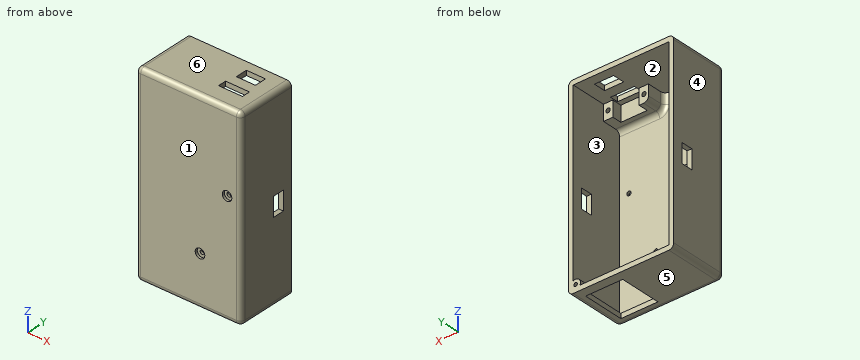
from build123d import *
from build123d.topology import SkipClean

# Parameters (mm, degrees)
SKETCH_1_W           = 44
SKETCH_1_H           = 81
EXTRUDE_1_DEPTH      = 25
SHELL_1_T            = -2
FILLET_1_R           = 2
SKETCH_2_R           = 0.8
SKETCH_2_R_2         = 0.9
CUT_EXTRUDE_1_DEPTH  = 24
SKETCH_3_R           = 1.25
CUT_EXTRUDE_2_DEPTH  = 24
SKETCH_4_R           = 6
EXTRUDE_2_DEPTH      = 2
CUT_EXTRUDE_START    = -13.2
SKETCH_6_R           = 1.25
CUT_EXTRUDE_4_DEPTH  = 13.2
SKETCH_7_W           = 15.5
SKETCH_7_H           = 17.5
CUT_EXTRUDE_5_DEPTH  = 13.2
SKETCH_9_W           = 18.8
SKETCH_9_H           = 6.5
SKETCH_9_R           = 0.9
EXTRUDE_3_DEPTH      = 8
SKETCH_11_W          = 11
SKETCH_11_H          = 6.5
CUT_EXTRUDE_6_DEPTH  = 4
SKETCH_12_W          = 10
SKETCH_12_H          = 3.5
CUT_EXTRUDE_7_DEPTH  = 4
FILLET_2_R           = 2
EXTRUDE_START        = -1
SKETCH_14_R          = 1.25
EXTRUDE_4_DEPTH      = 1
SKETCH_15_R          = 2
CUT_EXTRUDE_8_DEPTH  = 1
SKETCH_16_W          = 8
SKETCH_16_H          = 5
CUT_EXTRUDE_9_DEPTH  = 59
SKETCH_17_R          = 2
EXTRUDE_5_DEPTH      = 3
SKETCH_18_R          = 0.75
CUT_EXTRUDE_10_DEPTH = 3
FILLET_3_R           = 2
SKETCH_19_W          = 8
SKETCH_19_H          = 5
CUT_EXTRUDE_11_DEPTH = 3


with BuildPart() as part:
    # 草图1 → 凸台-拉伸1 (new body)
    with BuildSketch(Plane(origin=(0, 0, 0), x_dir=(1, 0, 0), z_dir=(0, 1, 0))):
        with Locations((0, -2.5)):
            Rectangle(SKETCH_1_W, SKETCH_1_H)
    extrude(amount=EXTRUDE_1_DEPTH)

    # 抽壳1
    shell_1_openings = [part.faces().sort_by_distance(p)[0] for p in [
        (0, 25, 2.5),
    ]]
    offset(amount=SHELL_1_T, openings=shell_1_openings, kind=Kind.INTERSECTION)

    # 圆角1
    fillet_1_edges = [part.edges().sort_by_distance(p)[0] for p in [
        (0, 0, -38),
        (22, 0, 2.5),
        (0, 0, 43),
        (-22, 0, 2.5),
        (-22, 12.5, -38),
        (22, 12.5, -38),
        (22, 12.5, 43),
        (-22, 12.5, 43),
    ]]
    fillet(fillet_1_edges, radius=FILLET_1_R)

    # 草图2 → 切除-拉伸1 (cut)
    with BuildSketch(Plane(origin=(0, 2, 0), x_dir=(1, 0, 0), z_dir=(0, 1, 0))):
        with Locations(Location((4.8, 16.9, 0), (0, 0, 270))):
            Circle(SKETCH_2_R)
        with Locations(Location((16.1, -9.5, 0), (0, 0, 270))):
            Circle(SKETCH_2_R_2)
    extrude(amount=-CUT_EXTRUDE_1_DEPTH, mode=Mode.SUBTRACT)

    # 草图3 → 切除-拉伸2 (cut)
    with BuildSketch(Plane(origin=(0, 2, 0), x_dir=(1, 0, 0), z_dir=(0, 1, 0))):
        with Locations(Location((-9.5, -3, 0), (0, 0, 270))):
            Circle(SKETCH_3_R)
    extrude(amount=-CUT_EXTRUDE_2_DEPTH, mode=Mode.SUBTRACT)

    # 草图4 → 凸台-拉伸2 (add)
    with BuildSketch(Plane(origin=(0, 2, 0), x_dir=(1, 0, 0), z_dir=(0, 1, 0))):
        with Locations(Location((-9.5, -3, 0), (0, 0, 270))):
            Circle(SKETCH_4_R)
    extrude(amount=EXTRUDE_2_DEPTH)

    # 草图6 → 切除-拉伸4 (cut)
    with BuildSketch(Plane.XZ.offset(CUT_EXTRUDE_START)):
        with Locations(Location((-9.5, 3, 0), (0, 0, 90))):
            Circle(SKETCH_6_R)
    extrude(amount=CUT_EXTRUDE_4_DEPTH, mode=Mode.SUBTRACT)

    # 草图7 → 切除-拉伸5 (cut)
    with BuildSketch(Plane(origin=(0, 0, -38), x_dir=(-1, 0, 0), z_dir=(0, 0, -1))):
        with Locations((-10.25, 12.5)):
            Rectangle(SKETCH_7_W, SKETCH_7_H)
    extrude(amount=-CUT_EXTRUDE_5_DEPTH, mode=Mode.SUBTRACT)

    # 草图9 → 凸台-拉伸3 (add)
    with BuildSketch(Plane(origin=(0, 2, 0), x_dir=(1, 0, 0), z_dir=(0, 1, 0))):
        with Locations((10.6, -37.75)):
            Rectangle(SKETCH_9_W, SKETCH_9_H)
        with Locations(Location((18.1, -37.9, 0), (0, 0, 270))):
            Circle(SKETCH_9_R, mode=Mode.SUBTRACT)
        with Locations(Location((3.1, -37.9, 0), (0, 0, 270))):
            Circle(SKETCH_9_R, mode=Mode.SUBTRACT)
    extrude(amount=EXTRUDE_3_DEPTH)

    # 草图11 → 切除-拉伸6 (cut)
    with BuildSketch(Plane(origin=(0, 10, 0), x_dir=(1, 0, 0), z_dir=(0, 1, 0))):
        with Locations((10.6, -37.75)):
            Rectangle(SKETCH_11_W, SKETCH_11_H)
    extrude(amount=-CUT_EXTRUDE_6_DEPTH, mode=Mode.SUBTRACT)

    # 草图12 → 切除-拉伸7 (cut)
    with BuildSketch(Plane.XY.offset(43)):
        with Locations((10.6, 10)):
            Rectangle(SKETCH_12_W, SKETCH_12_H)
    extrude(amount=-CUT_EXTRUDE_7_DEPTH, mode=Mode.SUBTRACT)

    # 圆角2
    fillet_2_edges = [part.edges().sort_by_distance(p)[0] for p in [
        (10.6, 2, 34.5),
        (1.2, 2, 37.75),
        (1.2, 6, 34.5),
    ]]
    fillet(fillet_2_edges, radius=FILLET_2_R)

    # 草图14 → 凸台-拉伸4 (add)
    with BuildSketch(Plane.XZ.offset(EXTRUDE_START)):
        with Locations(Location((-9.5, 3, 0), (0, 0, 90))):
            Circle(SKETCH_14_R)
    extrude(amount=EXTRUDE_4_DEPTH)

    # 草图15 → 切除-拉伸8 (cut)
    with BuildSketch(Plane.XZ):
        with Locations(Location((16.1, 9.5, 0), (0, 0, 270))):
            Circle(SKETCH_15_R)
        with Locations(Location((4.8, -16.9, 0), (0, 0, 270))):
            Circle(SKETCH_15_R)
    extrude(amount=-CUT_EXTRUDE_8_DEPTH, mode=Mode.SUBTRACT)

    # 草图16 → 切除-拉伸9 (cut)
    with BuildSketch(Plane.ZY.offset(22)):
        with Locations((0, 18.5)):
            Rectangle(SKETCH_16_W, SKETCH_16_H)
    extrude(amount=-CUT_EXTRUDE_9_DEPTH, mode=Mode.SUBTRACT)

    # 草图17 → 凸台-拉伸5 (add)
    with BuildSketch(Plane(origin=(0, 25, 0), x_dir=(1, 0, 0), z_dir=(0, 1, 0))):
        with Locations((19, 35)):
            Circle(SKETCH_17_R)
    extrude(amount=-EXTRUDE_5_DEPTH)

    # 草图18 → 切除-拉伸10 (cut)
    with BuildSketch(Plane(origin=(0, 25, 0), x_dir=(1, 0, 0), z_dir=(0, 1, 0))):
        with Locations(Location((19, 35, 0), (0, 0, 270))):
            Circle(SKETCH_18_R)
    extrude(amount=-CUT_EXTRUDE_10_DEPTH, mode=Mode.SUBTRACT)

    # 圆角3
    # the kernel refuses this fillet: 2 mm, written as the material it adds along each edge
    with BuildSketch(Plane(origin=(12.267949192, 22, -36), x_dir=(0, -1, 0), z_dir=(1, 0, 0))) as fillet_3_piece_1_section:
        with BuildLine():
            CenterArc((FILLET_3_R, -FILLET_3_R), FILLET_3_R, 90, 90)
            Line((0, -FILLET_3_R), (0, 0))
            Line((0, 0), (FILLET_3_R, 0))
        make_face()
    fillet_3_piece_1 = extrude(amount=7.732050808, mode=Mode.PRIVATE)
    fillet_3_piece_1 = fillet_3_piece_1 & Plane(origin=(19, 21.743486993, -35), x_dir=(1, 0, 0), z_dir=(0, 1, 0)) * Cylinder(2, 24, mode=Mode.PRIVATE)
    fillet_3_piece_1 = split(fillet_3_piece_1, bisect_by=Plane(origin=(18, 21.743486993, -35.418577815), z_dir=(-1, 0, 0)), keep=Keep.TOP, mode=Mode.PRIVATE)
    fillet_3_piece_1 = split(fillet_3_piece_1, bisect_by=Plane(origin=(17.546708028, 21.25, -35.418577815), z_dir=(0, 1, 0)), keep=Keep.TOP, mode=Mode.PRIVATE)
    add(fillet_3_piece_1)
    with BuildSketch(Plane(origin=(12.267949192, 22, -36), x_dir=(0, -1, 0), z_dir=(1, 0, 0))) as fillet_3_piece_2_section:
        with BuildLine():
            CenterArc((FILLET_3_R, -FILLET_3_R), FILLET_3_R, 90, 90)
            Line((0, -FILLET_3_R), (0, 0))
            Line((0, 0), (FILLET_3_R, 0))
        make_face()
    fillet_3_piece_2 = extrude(amount=7.732050808, mode=Mode.PRIVATE)
    fillet_3_piece_2 = split(fillet_3_piece_2, bisect_by=Plane(origin=(18, 20.864048259, -35.911747477), z_dir=(1, 0, 0)), keep=Keep.TOP, mode=Mode.PRIVATE)
    fillet_3_piece_2 = split(fillet_3_piece_2, bisect_by=Plane(origin=(18.99999999, 21.25, -35.911747477), z_dir=(0, -1, 0)), keep=Keep.TOP, mode=Mode.PRIVATE)
    fillet_3_piece_2 = fillet_3_piece_2 - Plane(origin=(19, 20.864048259, -35), x_dir=(0, 0, 1), z_dir=(0, 1, 0)) * Cylinder(0.75, 24, mode=Mode.PRIVATE)
    add(fillet_3_piece_2)
    with BuildSketch(Plane(origin=(12.267949192, 22, -36), x_dir=(0, -1, 0), z_dir=(1, 0, 0))) as fillet_3_piece_3_section:
        with BuildLine():
            CenterArc((FILLET_3_R, -FILLET_3_R), FILLET_3_R, 90, 90)
            Line((0, -FILLET_3_R), (0, 0))
            Line((0, 0), (FILLET_3_R, 0))
        make_face()
    fillet_3_piece_3 = extrude(amount=7.732050808, mode=Mode.PRIVATE)
    fillet_3_piece_3 = split(fillet_3_piece_3, bisect_by=Plane(origin=(18, 21.475531477, -35.364676357), z_dir=(1, 0, 0)), keep=Keep.TOP, mode=Mode.PRIVATE)
    fillet_3_piece_3 = split(fillet_3_piece_3, bisect_by=Plane(origin=(19.666666667, 21.25, -35.364676357), z_dir=(0, 1, 0)), keep=Keep.TOP, mode=Mode.PRIVATE)
    fillet_3_piece_3 = fillet_3_piece_3 - Plane(origin=(19, 21.475531477, -35), x_dir=(0, 0, 1), z_dir=(0, 1, 0)) * Cylinder(0.75, 24, mode=Mode.PRIVATE)
    add(fillet_3_piece_3)
    with BuildSketch(Plane(origin=(12.267949192, 22, -36), x_dir=(0, -1, 0), z_dir=(1, 0, 0))) as fillet_3_piece_4_section:
        with BuildLine():
            CenterArc((FILLET_3_R, -FILLET_3_R), FILLET_3_R, 90, 90)
            Line((0, -FILLET_3_R), (0, 0))
            Line((0, 0), (FILLET_3_R, 0))
        make_face()
    fillet_3_piece_4 = extrude(amount=12.732050808, mode=Mode.PRIVATE)
    fillet_3_piece_4 = split(fillet_3_piece_4, bisect_by=Plane(origin=(20, 20.885178509, -35.897350533), z_dir=(1, 0, 0)), keep=Keep.TOP, mode=Mode.PRIVATE)
    fillet_3_piece_4 = fillet_3_piece_4 & Plane(origin=(19, 20.885178509, -35), x_dir=(1, 0, 0), z_dir=(0, 1, 0)) * Cylinder(2, 34, mode=Mode.PRIVATE)
    fillet_3_piece_4 = split(fillet_3_piece_4, bisect_by=Plane(origin=(20.391607497, 21.25, -35.897350533), z_dir=(0, -1, 0)), keep=Keep.TOP, mode=Mode.PRIVATE)
    add(fillet_3_piece_4)
    with BuildSketch(Plane(origin=(12.267949192, 22, -36), x_dir=(0, -1, 0), z_dir=(1, 0, 0))) as fillet_3_piece_5_section:
        with BuildLine():
            CenterArc((FILLET_3_R, -FILLET_3_R), FILLET_3_R, 90, 90)
            Line((0, -FILLET_3_R), (0, 0))
            Line((0, 0), (FILLET_3_R, 0))
        make_face()
    fillet_3_piece_5 = extrude(amount=12.732050808, mode=Mode.PRIVATE)
    fillet_3_piece_5 = split(fillet_3_piece_5, bisect_by=Plane(origin=(20, 21.743487033, -35.418577693), z_dir=(1, 0, 0)), keep=Keep.TOP, mode=Mode.PRIVATE)
    fillet_3_piece_5 = fillet_3_piece_5 & Plane(origin=(19, 21.743487033, -35), x_dir=(1, 0, 0), z_dir=(0, 1, 0)) * Cylinder(2, 34, mode=Mode.PRIVATE)
    fillet_3_piece_5 = split(fillet_3_piece_5, bisect_by=Plane(origin=(20.45329205, 21.25, -35.418577693), z_dir=(0, 1, 0)), keep=Keep.TOP, mode=Mode.PRIVATE)
    add(fillet_3_piece_5)
    with BuildSketch(Plane(origin=(20, 22, -41), x_dir=(0, -1, 0), z_dir=(0, 0, 1))) as fillet_3_piece_6_section:
        with BuildLine():
            CenterArc((FILLET_3_R, -FILLET_3_R), FILLET_3_R, 90, 90)
            Line((0, -FILLET_3_R), (0, 0))
            Line((0, 0), (FILLET_3_R, 0))
        make_face()
    fillet_3_piece_6 = extrude(amount=12.732050808, mode=Mode.PRIVATE)
    fillet_3_piece_6 = fillet_3_piece_6 & Plane(origin=(19, 21.575046731, -35), x_dir=(1, 0, 0), z_dir=(0, 1, 0)) * Cylinder(2, 34, mode=Mode.PRIVATE)
    fillet_3_piece_6 = fillet_3_piece_6 - Plane(origin=(19, 21.575046731, -35), x_dir=(0, 0, 1), z_dir=(0, 1, 0)) * Cylinder(0.75, 34, mode=Mode.PRIVATE)
    add(fillet_3_piece_6)

    # 草图19 → 切除-拉伸11 (cut)
    with SkipClean():  # the faces are left unmerged after this step: merging them gives an invalid solid
        with BuildSketch(Plane.XY.offset(43)):
            with Locations((10.5, 18.5)):
                Rectangle(SKETCH_19_W, SKETCH_19_H)
        extrude(amount=-CUT_EXTRUDE_11_DEPTH, mode=Mode.SUBTRACT)


solid = part.part
Geometry check sheet. Reference: the model listing, model coordinates, mm. Face numbers are marked on the shaded views. A direction names the side the tool comes from. Round coordinates to 2 decimals unless told otherwise and drop trailing zeros. Write each loop counter-clockwise with the first axis right and the second up, starting at its lowest first coordinate (ties: lowest second). Pieces come first, ordered by that corner, then holes. Notation, with made-up numbers: (58.25, -34) - (94.25, -34) arc R25 cw to (94.25, -6) - close; hole circle Ø10 at (29.25, -7.5). An arc over 180 degrees is marked (long way). One line per item, written item: value.
1. Mould release check, pull along Z, two halves, no side actions. Record for the marked faces 3, 4, 5 and 6: released by +Z, released by -Z, zero draft, split by the parting line, or undercut.
The answers:
face 3: undercut
face 4: zero draft
face 5: released by -Z
face 6: released by +Z
2. Scan lines: L1, parallel to X at y = 22.9, z = -35; L2, parallel to Z at x = 19, y = 23.4; L3, parallel to X at y = 8.25, z = 37.9. Record each from-to range of solid material in increasing order.
The answers:
L1: x = -22 to -20, 17 to 18.25, 19.75 to 22
L2: z = -38 to -35.75, -34.25 to -33, 41 to 43
L3: x = -22 to -20, 1.2 to 2.2, 4 to 5.1, 16.1 to 17.2, 19 to 22
3. Cross-section at C-C on z = -16.9. Record the boundary of the cut face in (x, y).
The answers:
outline: (-22, 2) arc R2 ccw to (-20, 0) - (2.8, 0) - (2.8, 1) - (4, 1) - (4, 2) - (-20, 2) - (-20, 25) - (-22, 25) - close; (5.6, 1) - (6.8, 1) - (6.8, 0) - (20, 0) arc R2 ccw to (22, 2) - (22, 25) - (20, 25) - (20, 2) - (5.6, 2) - close
4. Set-up check for the marked faces 1 and 2: record each of +Z, -Z, +X, -X, +Y, -Y from which the full face is reachable in a straight line by a thin tool's end or side.
The answers:
face 1: +Z, -Z, +X, -X, -Y
face 2: +Y
5. Cross-section at B-B on x = 12. Record the boundary of the cut face in (y, z), and give its area (3 significant figures).
The answers:
outline: (0, -36) arc R2 ccw to (2, -38) - (3.75, -38) - (3.75, -36) - (2, -36) - (2, 32.5) arc R2 cw to (4, 34.5) - (6, 34.5) - (6, 41) - (8.25, 41) - (8.25, 43) - (2, 43) arc R2 ccw to (0, 41) - close; (11.75, 41) - (16, 41) - (16, 43) - (11.75, 43) - close; (21, 41) - (25, 41) - (25, 43) - (21, 43) - close; (21.25, -38) - (25, -38) - (25, -36) - (21.25, -36) - close
area: 227 mm^2
6. Cross-section at D-D on z = 37.9. Record the boundary of the cut face in (x, y), and give its area (3 significant figures).
The answers:
outline: (-22, 2) arc R2 ccw to (-20, 0) - (20, 0) arc R2 ccw to (22, 2) - (22, 25) - (20, 25) - (20, 10) - (19, 10) - (19, 2) - (17.2, 2) - (17.2, 10) - (16.1, 10) - (16.1, 6) - (5.1, 6) - (5.1, 10) - (4, 10) - (4, 2) - (2.2, 2) - (2.2, 10) - (1.2, 10) - (1.2, 4) arc R2 cw to (-0.8, 2) - (-20, 2) - (-20, 25) - (-22, 25) - close
area: 257 mm^2
7. Depth check by flat-ended pin: pin 1 Ø0.6 at (x, z) = (-21, 0) entering from -Y; pin 2 Ø1.6 at (y, z) = (12.5, -37) entering from +X; pin 3 Ø6 at (x, z) = (0, 25) entering from +Y; pin 4 Ø1 at (x, z) = (4.8, -16.9) entering from +Y. Enter the tip coordinate at first touch or a pass-through.
The answers:
pin 1: stops at y = 0.13
pin 2: stops at x = 21.99
pin 3: stops at y = 2
pin 4: passes through
8. Cross-section at A-A on y = 18.5. Record the boundary of the cut face in (x, z).
The answers:
outline: (-22, -36) arc R2 ccw to (-20, -38) - (2.5, -38) - (2.5, -36) - (-20, -36) - (-20, -4) - (-22, -4) - close; (-22, 4) - (-20, 4) - (-20, 41) - (6.5, 41) - (6.5, 43) - (-20, 43) arc R2 ccw to (-22, 41) - close; (14.5, 41) - (20, 41) - (20, 4) - (22, 4) - (22, 41) arc R2 ccw to (20, 43) - (14.5, 43) - close; (18, -38) - (20, -38) arc R2 ccw to (22, -36) - (22, -4) - (20, -4) - (20, -36) - (18, -36) - close
